Can you work these out from the model? Positions are in its coordinate system, mm. A direction names the side the tool comes from. Give positions to 0.01 mm unless a question says otherwise; leave off trailing zeros. Loops run counter-clockwise (first coordinate to the right, second up) from the corner with the lowest first, then second, coordinate; pieces in that order, holes last. Notation, with made-up numbers: M 52,-8 L 88,-8 A17 cw 88,7 Z; hole C 84.5,72.5 d7. An arc over 180 degrees is marked long. Put each result on its own line as item: value. Start each with the question number.
1) Imagine slicing it at C-C (z = -111). Write out the boundary of the cut face in (x, y) (3 decimals), then the cut area to 3 significant figures.
2) For P1, Ø17, axis at x = 203.2, z = -244.475, coming from the +Y side; P2, Ø2, axis at x = 7.5, y = 8.5, coming from the -Z side (3 decimals); P3, Ø3, axis at x = 247.5, y = 17, coming from the +Z side (3 decimals), each with a flat end and sliding along its axis, tell me the tip position at first contact or that it passes through.
3) Imagine slicing it at B-B (x = 109.5). Write out the boundary of the cut face in (y, z) (3 decimals), then the cut area to 3 significant figures.
4) Imagine slicing it at A-A (x = 50.8). Write out the boundary of the cut face in (y, z) (3 decimals), then the cut area to 3 significant figures.
5) For faces 5 (the flat face through (243.713, 13, -246)), 6 (the flat face through (28.575, 13, -128)), 7 (the flat face through (7, 13, -238.125)), which set-ups out of +Z, -Z, +X, -X, +Y, -Y let a thin tool reach every point of the face, with its end or its side?
6) Please list where these lines run through material, in increasing order: line 1 along Z through (x, y) = (203.2, 15.25) (3 decimals); line 2 along Z through (x, y) = (57, 6.25) (3 decimals); line 3 along X through (y, z) = (14.25, -57) (3 decimals). Write a range as from..to.
7) If we mould it in two halves opening along X, with no side actions, what happens to faces 1 (the flat face through (249, 13, -238.125)), 2 (the cylindrical face through (53.673, 12.522, -237.547)), 3 (the flat face through (10.287, 13, -246)), 4 (the flat face through (254, 13, -125))? For each: +X half, -X half, draft (parallel to the pull), parting line (faces both ways), or undercut.
8) Imagine slicing it at D-D (y = 6.25). Write out the boundary of the cut face in (x, z) (3 decimals), then the cut area to 3 significant figures.
Autodesk Inventor part; units mm, degrees
ref_plane "YZ Plane" through (0, 0, 0) normal (1, 0, 0) x (0, 1, 0)
ref_plane "XZ Plane" through (0, 0, 0) normal (0, 1, 0) x (-1, 0, 0)
ref_plane "XY Plane" through (0, 0, 0) normal (0, 0, 1) x (1, 0, 0)
sketch "Sketch1" plane through (0, 0, 0) normal (0, 1, 0) x (-1, 0, 0)
  line L0 (0, 0) -> (-254, 0)
  line L1 (-254, 0) -> (-254, -254)
  line L2 (-254, -254) -> (0, -254)
  line L3 (0, -254) -> (0, 0)
  line L4 (0, -15.875) -> (-10.287, -15.875)
  line L5 (-10.287, -15.875) -> (-10.287, 0)
  line L6 (-243.713, 0) -> (-243.713, -15.875)
  line L7 (-243.713, -15.875) -> (-254, -15.875)
  line L8 (-243.713, -254) -> (-243.713, -238.125)
  line L9 (-243.713, -238.125) -> (-254, -238.125)
  line L10 (-10.287, -254) -> (-10.287, -238.125)
  line L11 (-10.287, -238.125) -> (0, -238.125)
  dimension "d0" = 254
  dimension "d1" = 254
  dimension "d13" = 10.287
  dimension "d14" = 10.287
  dimension "d15" = 15.875
  dimension "d16" = 15.875
extrude "Extrusion1" add sketch "Sketch1" along normal blind 25.4 contours L5 L4 L3 L11 L10 L2 L8 L9 L1 L7 L6 L0
sketch "Sketch2" plane through (0, 25.4, 0) normal (0, 1, 0) x (1, 0, 0)
  line L0 (28.575, 28.575) -> (225.425, 28.575)
  line L1 (225.425, 28.575) -> (225.425, 225.425)
  line L2 (225.425, 225.425) -> (28.575, 225.425)
  line L3 (28.575, 225.425) -> (28.575, 28.575)
  line L4 (0, 15.875) -> (10.287, 15.875)
  line L5 (10.287, 15.875) -> (10.287, 0)
  line L6 (10.287, 0) -> (243.713, 0)
  line L7 (243.713, 0) -> (243.713, 15.875)
  line L8 (243.713, 15.875) -> (254, 15.875)
  line L9 (254, 15.875) -> (254, 238.125)
  line L10 (254, 238.125) -> (243.713, 238.125)
  line L11 (243.713, 238.125) -> (243.713, 254)
  line L12 (243.713, 254) -> (10.287, 254)
  line L13 (10.287, 254) -> (10.287, 238.125)
  line L14 (10.287, 238.125) -> (0, 238.125)
  line L15 (0, 238.125) -> (0, 15.875)
  point P0 (0, 0)
  point P1 (127, 28.575)
  point P2 (127, 0)
  point P3 (28.575, 127)
  point P4 (0, 127)
  dimension "d9" = 196.85
  dimension "d10" = 196.85
extrude "Extrusion2" cut sketch "Sketch2" against normal through all contours L3 L2 L1 L0
sketch "Sketch3" plane through (0, 25.4, 0) normal (0, 1, 0) x (1, 0, 0)
  circle A0 centre (50.8, 9.525) radius 7.5
  circle A1 centre (50.8, 244.475) radius 7.5
  circle A2 centre (203.2, 244.475) radius 4
  circle A3 centre (203.2, 244.475) radius 7.5
  circle A4 centre (203.2, 9.525) radius 7.5
  point P0 (0, 0)
hole "Hole1" at (50.8, 25.4, -9.525) at (50.8, 25.4, -244.475) at (203.2, 25.4, -9.525) at (203.2, 25.4, -244.475) direction (0, -1, 0) diameter 15 end through all
chamfer "Chamfer1" distance 3.175 angle 45 1 edges at (0, 12.7, -238.125)
equation "\"d14\" = d13"
equation "\"d9\" = d10"
properties part number "Carriage Sheet"
Recorded:
1. outline: M 0,0 L 28.575,0 L 28.575,25.4 L 0,25.4 Z; M 225.425,0 L 254,0 L 254,25.4 L 225.425,25.4 Z
1. area: 1,450 mm²
2. P1: y = 25.4
2. P2: z = -238.125
2. P3: z = -15.875
3. outline: M 0,-254 L 25.4,-254 L 25.4,-225.425 L 0,-225.425 Z; M 0,-28.575 L 25.4,-28.575 L 25.4,0 L 0,0 Z
3. area: 1,450 mm²
4. outline: M 0,-254 L 25.4,-254 L 25.4,-251.975 L 0,-251.975 Z; M 0,-236.975 L 25.4,-236.975 L 25.4,-225.425 L 0,-225.425 Z; M 0,-28.575 L 25.4,-28.575 L 25.4,-17.025 L 0,-17.025 Z; M 0,-2.025 L 25.4,-2.025 L 25.4,0 L 0,0 Z
4. area: 690 mm²
5. face 5: -Z, +X, +Y, -Y
5. face 6: +Y, -Y
5. face 7: -Z, -X, +Y, -Y
6. line 1: -254..-251.975, -236.975..-225.425, -28.575..-17.025, -2.025..0
6. line 2: -254..-248.695, -240.255..-225.425, -28.575..-13.745, -5.305..0
6. line 3: 0..28.575, 225.425..254
7. face 1: draft
7. face 2: undercut
7. face 3: -X half
7. face 4: +X half
8. outline: M 0,-234.95 L 3.175,-238.125 L 10.287,-238.125 L 10.287,-254 L 243.713,-254 L 243.713,-238.125 L 254,-238.125 L 254,-15.875 L 243.713,-15.875 L 243.713,0 L 10.287,0 L 10.287,-15.875 L 0,-15.875 Z; hole M 28.575,-225.425 L 225.425,-225.425 L 225.425,-28.575 L 28.575,-28.575 Z; hole C 50.8,-244.475 d15; hole C 50.8,-9.525 d15; hole C 203.2,-244.475 d15; hole C 203.2,-9.525 d15
8. area: 24,400 mm²
